Design review of the part built by this model. Coordinates are the model's own, in mm. Coordinates: 2 decimals unless noted, no trailing zeros. Write each loop counter-clockwise with the first axis right and the second up, starting at its lowest first coordinate (ties: lowest second). Pieces come first, ordered by that corner, then holes. Notation, with made-up numbers: M -21.5,51 L -17.5,51 A32 ccw -17.5,88 Z; hole C 12.25,-26.5 d5. An arc over 180 degrees is marked long. Write item = value, one per line.
```python
from build123d import *

# Parameters (mm, degrees)
F2_R = 1.19999
F3_R = 1.5


# Not quite as in the source:
# - a fillet or chamfer is up to 0.001 mm smaller than in the source, because OpenCascade refuses the exact size


with BuildPart() as f1:
    # F0 (on Front) → F1 (revolve)
    with BuildSketch(Plane.XZ):
        with BuildLine():
            Line((0, 22.8), (0, 24))
            ThreePointArc((0, 24), (-13.8564064606, 16), (-13.8564064606, 0))
            Line((-13.8564064606, 0), (-12.451505933, 0))
            ThreePointArc((-12.451505933, 0), (-13.8946821516, 13.0968429353), (-4.325, 22.1539526282))
            ThreePointArc((-4.325, 22.1539526282), (-3.7282728081, 22.322708608), (-3.125, 22.4663186402))
            ThreePointArc((-3.125, 22.4663186402), (-1.571382214, 22.7163432257), (0, 22.8))
        make_face()
        with BuildLine():
            Line((-3.125, 17.9663186402), (-3.125, 22.4663186402))
            ThreePointArc((-3.125, 22.4663186402), (-3.7282728081, 22.322708608), (-4.325, 22.1539526282))
            Line((-4.325, 22.1539526282), (-4.325, 17.9663186402))
            Line((-4.325, 17.9663186402), (-3.125, 17.9663186402))
        make_face()
    revolve(axis=Axis((0, 0, 23.4), (0, 0, 1)))

    # F2 (radius 1.2 in the source; OpenCascade refuses exactly that, so slightly less here)
    f2_edges = [f1.edges().sort_by_distance(p)[0] for p in [
        (3.125, 0, 17.966319),
    ]]
    fillet(f2_edges, radius=F2_R)

    # F3
    f3_edges = [f1.edges().sort_by_distance(p)[0] for p in [
        (4.325, 0, 22.153953),
    ]]
    fillet(f3_edges, radius=F3_R)


solid = f1.part
```
Q1. Consider section A-A, the plane z = 3.25. State the section outline as (x, y) points, and give its area (3 significant figures).
Check result:
outline = C 0,0 d30.56; hole C 0,0 d28.03
area = 116 mm²
Q2. Wall thickness on line 1 (X direction, y = -6.5, z = 7); line 2 (Y direction, x = 0, z = 20.25) (3 decimals); line 3 (Y direction, x = 0, z = 20.1) (3 decimals): over which ranges is each line inside the solid? List them lowest first.
Check result:
line_1 = -14.59 to -13.26, 13.26 to 14.59
line_2 = -10.293 to -8.305, -4.354 to -3.125, 3.125 to 4.354, 8.305 to 10.293
line_3 = -10.469 to -8.522, -4.332 to -3.125, 3.125 to 4.332, 8.522 to 10.469
Q3. Consider section B-B, the plane y = 12.5. State the section outline as (x, z) points, and give its area (3 significant figures).
Check result:
outline = M -5.98,0 L 5.98,0 A9.99 ccw long Z; hole C 0,8 d15.85
area = 99.9 mm²
Q4. Consider section C-C, the plane x = 11.5. State the section outline as (y, z) points, and give its area (3 significant figures).
Check result:
outline = M -7.73,0 L -4.77,0 A9.32 cw long 4.77,0 L 7.73,0 A11.12 ccw long Z
area = 91.4 mm²
Q5. For P1, Ø6, axis at x = -13, z = 4.5, coming from the -Y side; P2, Ø12, axis at x = -5.5, y = 7, coming from the +Z side; P3, Ø4, axis at x = -4, y = -6.5, coming from the +Z side, all flat-tipped, find the tip position at first contact; note any pin that passes through.
Check result:
P1 = -12.1
P2 = 23.73
P3 = 22.98
